Source: three-view drawing plus pictorial views. Frame: mm from the lowest corner of the part. A direction names the side the tool comes from. Round coordinates to 2 decimals unless told otherwise and drop trailing zeros. Loops run counter-clockwise (first coordinate to the right, second up) from the corner with the lowest first, then second, coordinate; pieces in that order, holes last. Notation, with made-up numbers: (77, 81) -> (91, 81) arc R26 cw to (91, 96) -> close; hole circle Ø1 at (44.25, -26.5). An arc over 180 degrees is marked (long way). Answer as a JSON object with one key per item and string values. Group by question number.
Item 1: Section query A-A on y = 4.25. Return loops of the section in (x, z).
Item 2: Draft query along Z for the marked faces 3, 4, 5 and 6. Return one class per face: released by +Z, released by -Z, zero draft, split by the parting line, or undercut.
Item 3: Pin query (flat end, axial travel): pin 1 (0.5 mm diameter, centred on x = 3.5, z = 2.5, fed in from +Y); pin 2 (2 mm diameter, centred on y = 5, z = 1, fed in from -X) (1 decimal); pin 3 (0.5 mm diameter, centred on x = 1, y = 9.5, fed in from +Z). Return the tip coordinate at first contact, or that it passes through.
Item 4: Set-up query: the marked faces 1 and 2. Return all of +Z, -Z, +X, -X, +Y, -Y with unobstructed straight access to the full face (end or side cutting, diameter ignored); none if empty.
Item 5: Material intervals for line 1 (Y direction, x = 3, z = 2.8); line 2 (Z direction, x = 2.35, y = 2.25); line 3 (X direction, y = 4.75, z = 2.65), sorted ascending. Write a range as [from, to].
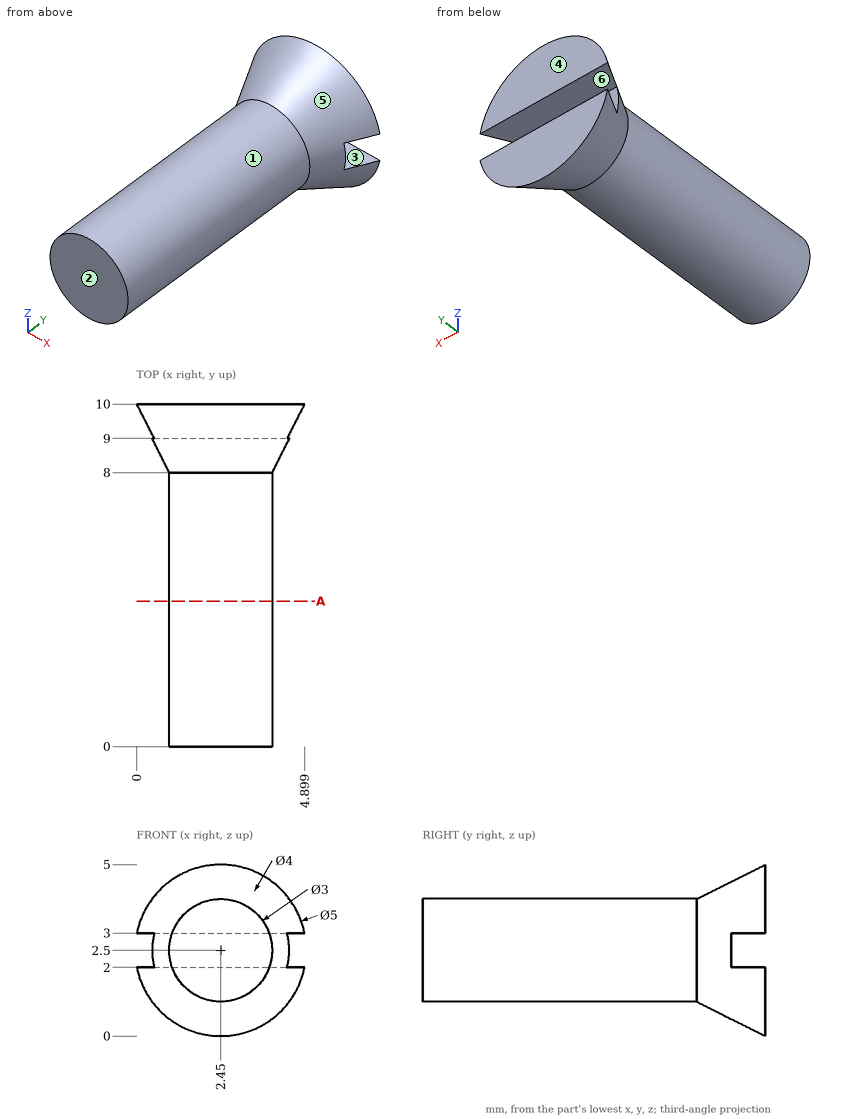
Solved:
{
 "1": {"outline": "circle Ø3 at (2.45, 2.5)"},
 "2": {"face 3": "undercut", "face 4": "zero draft", "face 5": "split by the parting line", "face 6": "undercut"},
 "3": {"pin 1": "y = 9", "pin 2": "x = 1", "pin 3": "z = 4.46"},
 "4": {"face 1": "-Y", "face 2": "+Z, -Z, +X, -X, -Y"},
 "5": {"line 1": "[0, 9]", "line 2": "[1, 4]", "line 3": "[0.96, 3.94]"}
}
